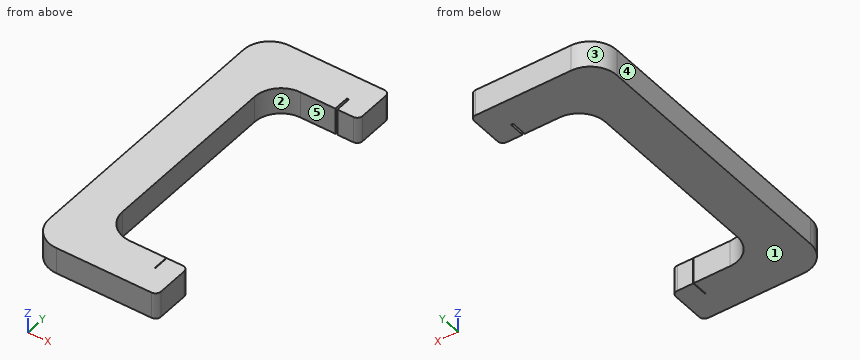
from build123d import *

# Parameters (mm, degrees)
BOSS_EXTRUDE1_DEPTH = 5
SKETCH3_W           = 0.1
SKETCH3_H           = 5
CUT_EXTRUDE1_DEPTH  = 3
SKETCH4_W           = 0.4
SKETCH4_H           = 5
CUT_EXTRUDE2_DEPTH  = 3


with BuildPart() as part:
    # Sketch1 → Boss-Extrude1 (new body)
    with BuildSketch(Plane.XY):
        with BuildLine():
            Line((0, 55), (0, 5))
            ThreePointArc((0, 5), (1.464466094, 1.464466094), (5, 0))
            Line((5, 0), (23, 0))
            ThreePointArc((23, 0), (23.707106781, 0.292893219), (24, 1))
            Line((24, 1), (24, 7))
            ThreePointArc((24, 7), (23.707106781, 7.707106781), (23, 8))
            Line((23, 8), (13, 8))
            ThreePointArc((13, 8), (9.464466094, 9.464466094), (8, 13))
            Line((8, 13), (8, 47))
            ThreePointArc((8, 47), (9.464466094, 50.535533906), (13, 52))
            Line((13, 52), (23, 52))
            ThreePointArc((23, 52), (23.707106781, 52.292893219), (24, 53))
            Line((24, 53), (24, 59))
            ThreePointArc((24, 59), (23.707106781, 59.707106781), (23, 60))
            Line((23, 60), (5, 60))
            ThreePointArc((5, 60), (1.464466094, 58.535533906), (0, 55))
        make_face()
    extrude(amount=BOSS_EXTRUDE1_DEPTH)

    # Sketch3 → Cut-Extrude1 (cut)
    with BuildSketch(Plane(origin=(0, 8, 0), x_dir=(1, 0, 0), z_dir=(0, 1, 0))):
        with Locations((19.95, -2.5)):
            Rectangle(SKETCH3_W, SKETCH3_H)
    extrude(amount=-CUT_EXTRUDE1_DEPTH, mode=Mode.SUBTRACT)

    # Sketch4 → Cut-Extrude2 (cut)
    with BuildSketch(Plane.XZ.offset(-52)):
        with Locations((19.8, 2.5)):
            Rectangle(SKETCH4_W, SKETCH4_H)
    extrude(amount=-CUT_EXTRUDE2_DEPTH, mode=Mode.SUBTRACT)


solid = part.part
The listing builds one solid part. Answer for the finished solid, in the listing's coordinates (mm). Face numbers are marked on the shaded views. A direction names the side the tool comes from. Round coordinates to 2 decimals unless told otherwise and drop trailing zeros. Order: outer loops, then holes, each group sorted by start corner. A loop starts at its lowest first (then second) coordinate and runs counter-clockwise, first axis right, second up. Notation, with made-up numbers: (-23.75, 39.25) - (-3.75, 39.25) arc R22 cw to (-3.75, 71.25) - close; hole circle Ø6 at (37, 28.5). An arc over 180 degrees is marked (long way). Write item = value, one per line. Start each with the question number.
1) Section B-B, the plane z = 3.1 is taken. Write down the section's boundary in (x, y), plus the area to 3 significant figures.
2) Section D-D, the plane y = 9 is taken. Write down the section's boundary in (x, z), plus the area to 3 significant figures.
3) Section A-A, the plane x = 22 is taken. Write down the section's boundary in (y, z).
4) Straight lines are drawn through the part: L1, parallel to Y at x = 15, z = 3.75; L2, parallel to X at y = 53, z = 4.25; L3, parallel to X at y = 52.5, z = 4.4. For each, find the intervals that lie inside material, in ascending order.
5) For the marked faces 4 and 5, determine the directions among +Z, -Z, +X, -X, +Y, -Y from which every point of the face is accessible in a straight line to the end or side of a thin tool.
6) Section C-C, the plane y = 37 is taken. Write down the section's boundary in (x, z).
7) For a pull along Y with two mould halves and no side action, classify the marked faces 1, 2 and 3 as released by +Y, released by -Y, zero draft, split by the parting line, or undercut.
Results list:
q1.outline = (0, 5) arc R5 ccw to (5, 0) - (23, 0) arc R1 ccw to (24, 1) - (24, 7) arc R1 ccw to (23, 8) - (20, 8) - (20, 5) - (19.9, 5) - (19.9, 8) - (13, 8) arc R5 cw to (8, 13) - (8, 47) arc R5 cw to (13, 52) - (19.6, 52) - (19.6, 55) - (20, 55) - (20, 52) - (23, 52) arc R1 ccw to (24, 53) - (24, 59) arc R1 ccw to (23, 60) - (5, 60) arc R5 ccw to (0, 55) - close
q1.area = 734 mm^2
q2.outline = (0, 0) - (10, 0) - (10, 5) - (0, 5) - close
q2.area = 50.0 mm^2
q3.outline = (0, 0) - (8, 0) - (8, 5) - (0, 5) - close; (52, 0) - (60, 0) - (60, 5) - (52, 5) - close
q4.L1 = 0 to 8, 52 to 60
q4.L2 = 0 to 19.6, 20 to 24
q4.L3 = 0 to 19.6, 20 to 23.87
q5.face_4 = +Z, -Z, -X, +Y, -Y
q5.face_5 = +Z, -Z, +X
q6.outline = (0, 0) - (8, 0) - (8, 5) - (0, 5) - close
q7.face_1 = zero draft
q7.face_2 = undercut
q7.face_3 = released by +Y
